CAD build for the part. Positions are in the model's coordinates, mm. Give positions to 0.01 mm unless a question says otherwise; leave off trailing zeros. Order: outer loops, then holes, each group sorted by start corner. A loop starts at its lowest first (then second) coordinate and runs counter-clockwise, first axis right, second up. Notation, with made-up numbers: M 64.5,-37 L 79.5,-37 A31 ccw 79.5,-4 Z; hole C 37.25,-17 d7. An arc over 180 degrees is marked long. Put each result on its own line as item: value. Start each with the question number.
1) Pin check, flat tip, straight feed: pin 1 (1.5 mm diameter, centred on x = -25.5, y = -1.5, fed in from +Z). Stop position of the tip, or through.
2) Cut at C-C (x = -50). Write the cut outline in (y, z).
3) Cut at D-D (y = -2.2). Give the number of separate pieces and of enclosed holes in the cut face, and give its area (3 significant figures).
4) Cut at A-A (z = -3.5). Write the cut outline in (x, y).
5) Cut at B-B (x = 100). Write the cut outline in (y, z), and give its area (3 significant figures).
6) Drill centre lines: line 1 (X direction, y = -1.05, z = -1); line 2 (Z direction, x = -80.5, y = -2.8); line 3 (Z direction, x = -74.5, y = -1.1). Where is each one in solid material? Low to high. Write a range as [from, to].
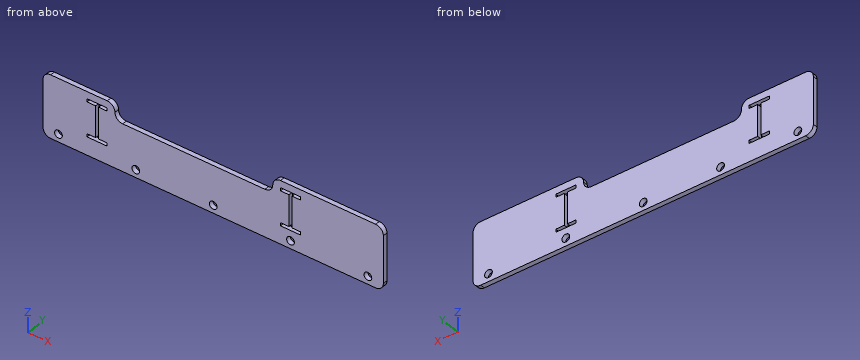
```python
from build123d import *

# Parameters (mm, degrees)
F0_R     = 2.5
F1_DEPTH = 3


with BuildPart() as f1:
    # F0 (on Front) → F1 (new body)
    with BuildSketch(Plane.XZ):
        with BuildLine():
            Line((-68.5, 20), (-105, 20))
            ThreePointArc((-105, 20), (-108.535534, 18.535534), (-110, 15))
            Line((-110, 15), (-110, -15))
            ThreePointArc((-110, -15), (-108.535534, -18.535534), (-105, -20))
            Line((-105, -20), (105, -20))
            ThreePointArc((105, -20), (108.535534, -18.535534), (110, -15))
            Line((110, -15), (110, 15))
            ThreePointArc((110, 15), (108.535534, 18.535534), (105, 20))
            Line((105, 20), (43.5, 20))
            ThreePointArc((43.5, 20), (39.964466, 18.535534), (38.5, 15))
            ThreePointArc((38.5, 15), (37.035534, 11.464466), (33.5, 10))
            Line((33.5, 10), (-58.5, 10))
            ThreePointArc((-58.5, 10), (-62.035534, 11.464466), (-63.5, 15))
            ThreePointArc((-63.5, 15), (-64.964466, 18.535534), (-68.5, 20))
        make_face()
        with Locations((-100, -15)):
            Circle(F0_R, mode=Mode.SUBTRACT)
        with Locations((-50, -15)):
            Circle(F0_R, mode=Mode.SUBTRACT)
        with Locations((0, -15)):
            Circle(F0_R, mode=Mode.SUBTRACT)
        with Locations((50, -15)):
            Circle(F0_R, mode=Mode.SUBTRACT)
        with Locations((100, -15)):
            Circle(F0_R, mode=Mode.SUBTRACT)
        Polygon((-81.5, 13.5), (-81.5, 15.5), (-68.5, 15.5), (-68.5, 13.5), (-74, 13.5), (-74, -6.5), (-68.5, -6.5), (-68.5, -8.5), (-81.5, -8.5), (-81.5, -6.5), (-76, -6.5), (-76, 13.5), align=None, mode=Mode.SUBTRACT)
        Polygon((43.5, -6.5), (49, -6.5), (49, 13.5), (43.5, 13.5), (43.5, 15.5), (56.5, 15.5), (56.5, 13.5), (51, 13.5), (51, -6.5), (56.5, -6.5), (56.5, -8.5), (43.5, -8.5), align=None, mode=Mode.SUBTRACT)
    extrude(amount=F1_DEPTH)


solid = f1.part
```
Solution:
1. pin 1: z = 10
2. outline: M -3,-20 L 0,-20 L 0,-17.5 L -3,-17.5 Z; M -3,-12.5 L 0,-12.5 L 0,10 L -3,10 Z
3. separate pieces: 1
3. enclosed holes: 7
3. area: 7,480 mm²
4. outline: M -110,-3 L -76,-3 L -76,0 L -110,0 Z; M -74,-3 L 49,-3 L 49,0 L -74,0 Z; M 51,-3 L 110,-3 L 110,0 L 51,0 Z
5. outline: M -3,-20 L 0,-20 L 0,-17.5 L -3,-17.5 Z; M -3,-12.5 L 0,-12.5 L 0,20 L -3,20 Z
5. area: 105 mm²
6. line 1: [-110, -76], [-74, 49], [51, 110]
6. line 2: [-20, -8.5], [-6.5, 13.5], [15.5, 20]
6. line 3: [-20, -8.5], [15.5, 20]
